from build123d import *

# Parameters (mm, degrees)
ESQUISSE1_R                  = 7.6
BOSS_EXTRU_1_DEPTH           = 20
ESQUISSE8_W                  = 22.8
ESQUISSE8_H                  = 20
BOSS_EXTRU_4_DEPTH           = 3
ESQUISSE2_W                  = 35
ESQUISSE2_H                  = 2.5
BOSS_EXTRU_2_DEPTH           = 12
ESQUISSE3_R                  = 2.6
ENL_V_MAT_EXTRU_1_DEPTH      = 3
ENL_V_MAT_EXTRU_1_DEPTH_BACK = 22
CHANFREIN1_SIZE              = 3.5
ESQUISSE4_W                  = 10
ESQUISSE4_H                  = 20
BOSS_EXTRU_3_DEPTH           = 13
ENL_V_MAT_EXTRU_2_DEPTH      = 10


with BuildPart() as part:
    # Esquisse1 → Boss.-Extru.1 (new body)
    with BuildSketch(Plane(origin=(0, 0, 0), x_dir=(1, 0, 0), z_dir=(0, 1, 0))):
        with BuildLine():
            Line((47, -20), (43, -20))
            ThreePointArc((43, -20), (37.343145751, -17.656854249), (35, -12))
            Line((35, -12), (35, -5))
            Line((35, -5), (-35, -5))
            Line((-35, -5), (-35, -12))
            ThreePointArc((-35, -12), (-37.343145751, -17.656854249), (-43, -20))
            Line((-43, -20), (-47, -20))
            ThreePointArc((-47, -20), (-52.656854249, -17.656854249), (-55, -12))
            Line((-55, -12), (-55, 0))
            Line((-55, 0), (55, 0))
            Line((55, 0), (55, -12))
            ThreePointArc((55, -12), (52.656854249, -17.656854249), (47, -20))
        make_face()
        with Locations((45, -10)):
            Circle(ESQUISSE1_R, mode=Mode.SUBTRACT)
        with Locations((-45, -10)):
            Circle(ESQUISSE1_R, mode=Mode.SUBTRACT)
    extrude(amount=BOSS_EXTRU_1_DEPTH)

    # Esquisse8 → Boss.-Extru.4 (add)
    with BuildSketch(Plane(origin=(0, 0, 0), x_dir=(-1, 0, 0), z_dir=(0, 0, -1))):
        with Locations((-20.6, 10)):
            Rectangle(ESQUISSE8_W, ESQUISSE8_H)
    extrude(amount=BOSS_EXTRU_4_DEPTH)

    # Esquisse2 → Boss.-Extru.2 (add)
    with BuildSketch(Plane(origin=(0, 0, 0), x_dir=(-1, 0, 0), z_dir=(0, 0, -1))):
        with Locations((-37.5, 18.75)):
            Rectangle(ESQUISSE2_W, ESQUISSE2_H)
        with Locations((-37.5, 1.25)):
            Rectangle(ESQUISSE2_W, ESQUISSE2_H)
    extrude(amount=BOSS_EXTRU_2_DEPTH)

    # Esquisse3 → Enlèv. mat.-Extru.1 (cut, two sides)
    with BuildSketch(Plane(origin=(0, 0, 0), x_dir=(-1, 0, 0), z_dir=(0, 0, -1))) as enl_v_mat_extru_1_sk:
        with Locations((-13.2, 10)):
            Circle(ESQUISSE3_R)
        with Locations((-28, 10)):
            Circle(ESQUISSE3_R)
    extrude(amount=ENL_V_MAT_EXTRU_1_DEPTH, mode=Mode.SUBTRACT)
    extrude(enl_v_mat_extru_1_sk.sketch, amount=-ENL_V_MAT_EXTRU_1_DEPTH_BACK, mode=Mode.SUBTRACT)

    # Chanfrein1
    chanfrein1_edges = [part.edges().sort_by_distance(p)[0] for p in [
        (15.8, 10, 5),
        (30.6, 10, 5),
    ]]
    chamfer(chanfrein1_edges, length=CHANFREIN1_SIZE)

    # Esquisse4 → Boss.-Extru.3 (add)
    with BuildSketch(Plane(origin=(0, 0, 0), x_dir=(0, 0, -1), z_dir=(1, 0, 0))):
        with Locations((-10, 10)):
            Rectangle(ESQUISSE4_W, ESQUISSE4_H)
    extrude(amount=-BOSS_EXTRU_3_DEPTH)

    # Esquisse7 → Enlèv. mat.-Extru.2 (cut)
    with BuildSketch(Plane.XY.offset(15)):
        with BuildLine():
            Line((-8.2, 20), (-6.5, 20))
            add(Edge.make_bspline(
                [(-6.5, 20), (-7.602205078, 16.366247775), (0.602205078, 10), (-7.602205078, 3.633752225), (-6.5, 0)],
                knots=[0, 0, 0, 0, 0.5, 1, 1, 1, 1], degree=3))
            Line((-6.5, 0), (-8.2, 0))
            add(Edge.make_bspline(
                [(-8.2, 20), (-9.302205078, 16.366247775), (-1.097794922, 10), (-9.302205078, 3.633752225), (-8.2, 0)],
                knots=[0, 0, 0, 0, 0.5, 1, 1, 1, 1], degree=3))
        make_face()
    extrude(amount=-ENL_V_MAT_EXTRU_2_DEPTH, mode=Mode.SUBTRACT)


solid = part.part
For this review, take the finished solid that the model builds, in its own axes (mm). A direction names the side the tool comes from. Give positions to 0.01 mm unless a question says otherwise; leave off trailing zeros. Order: outer loops, then holes, each group sorted by start corner. A loop starts at its lowest first (then second) coordinate and runs counter-clockwise, first axis right, second up. Notation, with made-up numbers: (-18.75, 31.25) -> (-13.75, 31.25) arc R25 cw to (-13.75, 63.25) -> close; hole circle Ø4 at (-8.5, 73.25). An arc over 180 degrees is marked (long way). Write item = value, one per line.
1) Insertion check: pin 1 (13.5 mm diameter, centred on x = 45, z = 10, fed in from -Y); pin 2 (2 mm diameter, centred on x = -3, y = 12.5, fed in from +Z); pin 3 (1 mm diameter, centred on x = 11.5, z = -3, fed in from -Y); pin 4 (7 mm diameter, centred on x = 28, y = 10, fed in from -Z). Each pin has a flat end and moves straight along its axis. Give the tip position at first contact, or say it passes through.
Findings:
pin_1 = through
pin_2 = 15
pin_3 = 0
pin_4 = -3
2) We need section C-C, the plane y = 10. Count the separate pieces of the cut face and the enclosed holes in it, and give its area (3 significant figures).
Findings:
separate_pieces = 3
enclosed_holes = 2
area = 806 mm^2
3) For faces 1 (the face through (45, 10, 20)), 2 (the face through (38, 2.5, -6)), 3 (the face through (13, 0, 4)), 4 (the face through (0, 10, 10)), 5 (the face through (-23, 10, 0)), list the 3-axis set-ups (+Z, -Z, +X, -X, +Y, -Y) from which the entire face can be reached by the end or side of a thin tool; tool diameter is ignored.
Findings:
face_1 = +Z, +X, -X, +Y, -Y
face_2 = -Z, +X
face_3 = +Z, -Z, +X, -X, -Y
face_4 = +Z, +Y, -Y
face_5 = -Z, -X, +Y, -Y
4) Draft analysis for pull direction X (two halves, no side actions). For faces 6 (the face through (52.25, 9.86, 7.72)), 7 (the face through (38, 17.5, -6)), 8 (the face through (20, 1, -7)), state which applies: pulls with the +X half, pulls with the -X half, needs draft (parallel to the pull), parting line crosses it, or undercut.
Findings:
face_6 = undercut
face_7 = needs draft
face_8 = pulls with the -X half
5) We need section D-D, the plane x = 45. Give the boundary of the cut face in (y, z), and give its area (3 significant figures).
Findings:
outline = (0, -12) -> (2.5, -12) -> (2.5, 0) -> (17.5, 0) -> (17.5, -12) -> (20, -12) -> (20, 2.4) -> (0, 2.4) -> close; (0, 17.6) -> (20, 17.6) -> (20, 20) -> (0, 20) -> close
area = 156 mm^2
6) We need section B-B, the plane z = -9. Give the boundary of the cut face in (x, y).
Findings:
outline = (20, 0) -> (55, 0) -> (55, 2.5) -> (20, 2.5) -> close; (20, 17.5) -> (55, 17.5) -> (55, 20) -> (20, 20) -> close
7) To check wall thickness, follow L1, parallel to Y at x = 28, z = 1.2; L2, parallel to X at y = 1.75, z = 15.5 (3 decimals); L3, parallel to X at y = 5.25, z = 10. State the ranges of each line that lie inside material, in increasing order. Write a range as from..to.
Findings:
L1 = 0..7.4, 12.6..20
L2 = -54.194..-50.245, -39.755..-35.806, 35.806..39.755, 50.245..54.194
L3 = -55..-52.6, -37.4..-35, -13..-7.07, -5.37..0, 35..37.4, 52.6..55
8) We need section A-A, the plane x = 13.2. Give the boundary of the cut face in (y, z).
Findings:
outline = (0, -3) -> (7.4, -3) -> (7.4, 1.5) -> (3.9, 5) -> (0, 5) -> close; (12.6, -3) -> (20, -3) -> (20, 5) -> (16.1, 5) -> (12.6, 1.5) -> close
